Could you check a few things on this drawing? It's one solid part, dimensions in mm from its lowest x, y, z. A direction names the side the tool comes from. Coordinates: 2 decimals unless noted, no trailing zeros. Order: outer loops, then holes, each group sorted by start corner. A loop starts at its lowest first (then second) coordinate and runs counter-clockwise, first axis right, second up. Notation, with made-up numbers: (38.25, -18) - (46.25, -18) arc R27 ccw to (46.25, 11) - close; hole circle Ø6 at (77.25, 36). An arc over 180 degrees is marked (long way). Answer in a Markdown table with one row per item. Add a question column.
Item 1: I want a section at C-C (y = 23). Please give me the cut outline in (x, z).
Item 2: I want a section at D-D (x = 41.5). Please give me the cut outline in (y, z).
Item 3: I want a section at B-B (x = 20). Please give me the cut outline in (y, z), plus the area to 3 significant figures.
Item 4: On a 3-axis mill with a long thin cutter (end or side, diameter ignored), from which of +Z, -Z, +X, -X, +Y, -Y can I reach the whole of each face in a straight line? I mean the marked faces 1, 2 and 3. Say none if no direction works.
Item 5: I want a section at A-A (z = 27.5). Please give me the cut outline in (x, y).
Item 6: Will these pins go through, and if not, where does the flat tip stop? pin 1 Ø2 at (x, y) = (104.5, 3) entering from +Z; pin 2 Ø11.5 at (x, z) = (20, 52.5) entering from +Y; pin 3 Ø1 at (x, z) = (23, 13.5) entering from -Y; pin 4 Ø12 at (y, z) = (18, 51) entering from +X.
Item 7: If I drill on line 1 along Z through (x, y) = (20, 13.5); line 2 along Z through (x, y) = (80, 19.5); line 3 along X through (y, z) = (5, 8.5), over which ranges is the centre line in solid material (lowest first)? Write a range as from..to.
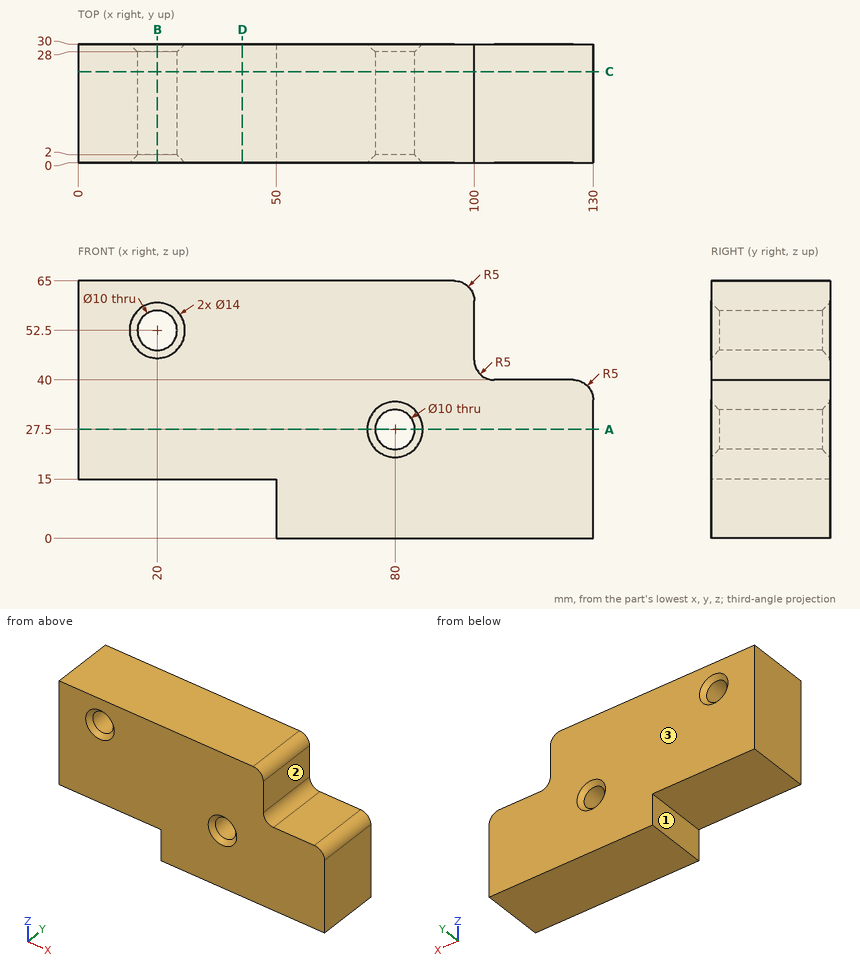
Values follow:
| question | item | result |
|---|---|---|
| 1 | outline | (0, 15) - (50, 15) - (50, 0) - (130, 0) - (130, 35) arc R5 ccw to (125, 40) - (105, 40) arc R5 cw to (100, 45) - (100, 60) arc R5 ccw to (95, 65) - (0, 65) - close; hole circle Ø10 at (20, 52.5); hole circle Ø10 at (80, 27.5) |
| 2 | outline | (0, 15) - (30, 15) - (30, 65) - (0, 65) - close |
| 3 | outline | (0, 15) - (30, 15) - (30, 45.5) - (28, 47.5) - (2, 47.5) - (0, 45.5) - close; (0, 59.5) - (2, 57.5) - (28, 57.5) - (30, 59.5) - (30, 65) - (0, 65) - close |
| 3 | area | 1,190 mm^2 |
| 4 | face 1 | -Z, -X, +Y, -Y |
| 4 | face 2 | +Z, +X, +Y, -Y |
| 4 | face 3 | +Z, -Z, +X, -X, +Y |
| 5 | outline | (0, 0) - (73, 0) - (75, 2) - (75, 28) - (73, 30) - (0, 30) - close; (85, 2) - (87, 0) - (130, 0) - (130, 30) - (87, 30) - (85, 28) - close |
| 6 | pin 1 | stops at z = 40.23 |
| 6 | pin 2 | stops at y = 28.75 |
| 6 | pin 3 | passes through |
| 6 | pin 4 | stops at x = 100 |
| 7 | line 1 | z = 15..47.5, 57.5..65 |
| 7 | line 2 | z = 0..22.5, 32.5..65 |
| 7 | line 3 | x = 50..130 |
